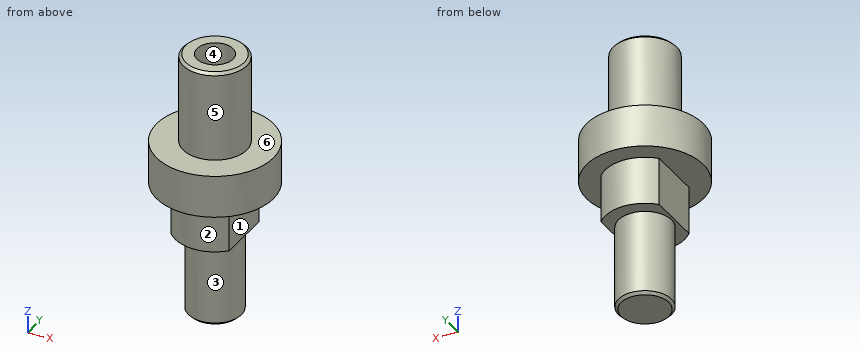
from build123d import *

# Parameters (mm, degrees)
SKETCH_2_OUTSIDE_W   = 35.778
SKETCH_2_OUTSIDE_H   = 35.778
SKETCH_2_OUTSIDE_W_2 = 11
SKETCH_2_OUTSIDE_H_2 = 17.627531483
CUT_EXTRUDE_1_DEPTH  = 9
M8X1_25_1_D          = 6.8
M8X1_25_1_DEPTH      = 19.75
M8X1_25_1_TIP        = 2.042926105
CHAMFER_1_SIZE       = 0.5


with BuildPart() as part:
    # 草图1 → 旋转1 (revolve)
    with BuildSketch(Plane(origin=(0, 0, 0), x_dir=(0, 0, -1), z_dir=(1, 0, 0)), mode=Mode.PRIVATE) as revolve_1_sk:
        Polygon((0, 6), (17, 6), (17, 11), (25, 11), (25, 7.5), (34, 7.5), (34, 5), (50, 5), (50, 0), (0, 0), align=None)
    revolve(revolve_1_sk.sketch.rotate(Axis((0, 0, -50), (0, 0, 1)), 90), axis=Axis((0, 0, -50), (0, 0, 1)))

    # 草图2 outside → 切除-拉伸1 (cut)
    with BuildSketch(Plane.XY.offset(-34)):
        Rectangle(SKETCH_2_OUTSIDE_W, SKETCH_2_OUTSIDE_H)
        with Locations((0, -0.228588755)):
            Rectangle(SKETCH_2_OUTSIDE_W_2, SKETCH_2_OUTSIDE_H_2, mode=Mode.SUBTRACT)
    extrude(amount=CUT_EXTRUDE_1_DEPTH, mode=Mode.SUBTRACT)

    # M8x1.25 螺纹孔1
    with Locations(Plane.XY):
        with Locations((0, 0)):
            Hole(M8X1_25_1_D / 2, depth=M8X1_25_1_DEPTH)
            with Locations((0, 0, -(M8X1_25_1_DEPTH + M8X1_25_1_TIP / 2))):  # 118° drill point
                Cone(0, M8X1_25_1_D / 2, M8X1_25_1_TIP, mode=Mode.SUBTRACT)

    # 倒角1
    chamfer_1_edges = [part.edges().sort_by_distance(p)[0] for p in [
        (6, 0, 0),
        (5, 0, -50),
    ]]
    chamfer(chamfer_1_edges, length=CHAMFER_1_SIZE)


solid = part.part
Can you work these out from the model? Positions are in its coordinate system, mm. Face numbers are marked on the shaded views. A direction names the side the tool comes from. Give positions to 0.01 mm unless a question says otherwise; leave off trailing zeros. Order: outer loops, then holes, each group sorted by start corner. A loop starts at its lowest first (then second) coordinate and runs counter-clockwise, first axis right, second up. Notation, with made-up numbers: M 16.25,-3.75 L 36.25,-3.75 A19 cw 36.25,32.25 Z; hole C 62.5,34 d8. An arc over 180 degrees is marked long. One line per item, written item: value.
Item 1: If we section it at C-C on z = -44: Write out the boundary of the cut face in (x, y).
Verdict:
outline: C 0,0 d10
Item 2: If we section it at D-D on z = -31.5: Write out the boundary of the cut face in (x, y).
Verdict:
outline: M -5.5,-5.1 A7.5 ccw 5.5,-5.1 L 5.5,5.1 A7.5 ccw -5.5,5.1 Z
Item 3: For pin 1 (6 mm diameter, centred on x = -3, y = -4, fed in from -Z); pin 2 (1.5 mm diameter, centred on x = 3.5, z = -7.5, fed in from +Y); pin 3 (7 mm diameter, centred on y = 2, z = -31, fed in from +X); pin 4 (7 mm diameter, centred on y = 0, z = -31, fed in from -X), each with a flat end and sliding along its axis, tell me the tip position at first contact or that it passes through.
Verdict:
pin 1: z = -50
pin 2: y = 5.33
pin 3: x = 5.5
pin 4: x = -5.5
Item 4: Please list where these lines run through material, in increasing order: line 1 (Y direction, x = 0, z = -14); line 2 (Z direction, x = 6.25, y = -3.75); line 3 (X direction, y = -2.5, z = -30).
Verdict:
line 1: -6 to -3.4, 3.4 to 6
line 2: -25 to -17
line 3: -5.5 to 5.5
Item 5: If we section it at A-A on z = -16: Write out the boundary of the cut face in (x, y).
Verdict:
outline: C 0,0 d12; hole C 0,0 d6.8
Item 6: If we section it at B-B on y = -6.75: Write out the boundary of the cut face in (x, z).
Verdict:
outline: M -8.69,-25 L -3.27,-25 L -3.27,-34 L 3.27,-34 L 3.27,-25 L 8.69,-25 L 8.69,-17 L -8.69,-17 Z
Item 7: For the marked faces 1, 2 and 3, which set-ups out of +Z, -Z, +X, -X, +Y, -Y let a thin tool reach every point of the face, with its end or its side?
Verdict:
face 1: -Z, +X, +Y, -Y
face 2: -Z, -Y
face 3: -Z
Item 8: If we mould it in two halves opening along Y, with no side actions, what happens to the marked faces 4, 5 and 6? For each: pulls with the +Y half, pulls with the -Y half, needs draft (parallel to the pull), parting line crosses it, or undercut.
Verdict:
face 4: undercut
face 5: parting line crosses it
face 6: needs draft
